CAD build for the part. Positions are in the model's coordinates, mm. A direction names the side the tool comes from. Give positions to 0.01 mm unless a question says otherwise; leave off trailing zeros. Write each loop counter-clockwise with the first axis right and the second up, starting at its lowest first coordinate (ties: lowest second). Pieces come first, ordered by that corner, then holes. Notation, with made-up numbers: (29.5, 68.25) - (81.5, 68.25) arc R23 ccw to (81.5, 104.25) - close; hole circle Ø7 at (69.25, -33). An arc over 180 degrees is marked (long way). Answer as a JSON object with one key per item and string values.
Autodesk Inventor part; units mm, degrees
ref_plane "YZ Plane" through (0, 0, 0) normal (1, 0, 0) x (0, 1, 0)
ref_plane "XZ Plane" through (0, 0, 0) normal (0, 1, 0) x (-1, 0, 0)
ref_plane "XY Plane" through (0, 0, 0) normal (0, 0, 1) x (1, 0, 0)
sketch "Sketch1" plane through (0, 0, 0) normal (1, 0, 0) x (0, 1, 0)
  line L0 (0, 9.5) -> (0, -9.5)
  line L1 (0, -9.5) -> (8, -9.5)
  line L2 (0, 9.5) -> (8, 9.5)
  line L3 (8, 9.5) -> (8, 14.5)
  line L4 (8, 14.5) -> (9.5, 14.5)
  line L5 (9.5, 14.5) -> (9.5, 10.5)
  line L6 (9.5, 10.5) -> (11.5, 10.5)
  line L7 (11.5, 10.5) -> (11.5, 16.5)
  line L8 (11.5, 16.5) -> (6, 16.5)
  line L9 (6, 16.5) -> (6, 11.5)
  line L10 (6, 11.5) -> (-3, 11.5)
  line L11 (-3, 11.5) -> (-4, 11.5)
  line L12 (-4, 11.5) -> (-4, 1)
  line L13 (0, 0) -> (3.5, 0)
  line L14 (0, -9.5) -> (8, -9.5)
  line L15 (8, -9.5) -> (8, -14.5)
  line L16 (8, -14.5) -> (9.5, -14.5)
  line L17 (9.5, -14.5) -> (9.5, -10.5)
  line L18 (11.5, -10.5) -> (11.5, -16.5)
  line L19 (11.5, -16.5) -> (6, -16.5)
  line L20 (6, -16.5) -> (6, -11.5)
  line L21 (6, -11.5) -> (-3, -11.5)
  line L22 (-3, -11.5) -> (-4, -11.5)
  line L23 (-4, -11.5) -> (-4, 1)
  line L24 (11.5, -10.5) -> (9.5, -10.5)
  point P0 (8.75, -16.5)
  point P1 (8.75, -14.5)
  dimension "d0" = 19
  dimension "d1" = 0
  dimension "d2" = 8
  dimension "d3" = 8
  dimension "d4" = 5
  dimension "d5" = 1.5
  dimension "d6" = 2
  dimension "d7" = 6
  dimension "d8" = 5.5
  dimension "d9" = 5
  dimension "d10" = 1
  dimension "d13" = 2
  dimension "d14" = 4
extrude "Extrusion1" add sketch "Sketch1" along normal blind 20
fillet "Fillet1" radius 5 2 edges at (10, 6, -11.5) (10, 6, 11.5)
chamfer "Chamfer1" distance 1 angle 45 12 edges at (20, 8, -12) (20, 8.75, -14.5) (20, 9.5, -12.5) (20, 8, 12) (20, 8.75, 14.5) (20, 9.5, 12.5) (0, 8, -12) (0, 8.75, -14.5) (0, 9.5, -12.5) (0, 8, 12) (0, 8.75, 14.5) (0, 9.5, 12.5)
sketch "Sketch2" plane through (0, 0, 9.5) normal (0, 1, 0) x (1, 0, 0)
  circle A0 centre (10, 9.5) radius 3
  line L0 (20, 19) -> (20, 0)
  line L1 (0, -7) -> (20, -7)
  point P0 (0, 9.5)
  dimension "d19" = 6
  dimension "d20" = 10
  dimension "d21" = 16.5
extrude "Extrusion2" cut sketch "Sketch2" against normal blind 20
chamfer "Chamfer2" distance 2.5 angle 45 1 edges at (7, 0, 0)
properties part number "Drziak_1"
(1) Saw through at D-D, the plane y = -1.5. Give the cut face in (x, z).
Answer key:
{"outline": "(0, -11.5) - (20, -11.5) - (20, 11.5) - (0, 11.5) - close; hole circle Ø8 at (10, 0)"}
(2) Pull direction Y, two halves, no side cores. Call faces 1 (the face through (10, 8, 12)), 2 (the face through (10.14, 4.5, 12.93)), 3 (the face through (10, 11, -10.5)): pulls with the +Y half, pulls with the -Y half, needs draft (parallel to the pull), parting line crosses it, or undercut.
Answer key:
{"face 1": "undercut", "face 2": "pulls with the -Y half", "face 3": "needs draft"}
(3) 3-axis set-ups, long thin cutter, end or side, ignore diameter. For faces 4 (the face through (0.5, 7.5, -12.5)), 5 (the face through (5, 0, 4)), 6 (the face through (10, -1, 11.5)), 7 (the face through (19.5, 7.5, -12.5)): which of +Z, -Z, +X, -X, +Y, -Y reach the whole face in a straight line?
Answer key:
{"face 4": "-X", "face 5": "+X, -X, +Y", "face 6": "+Z, +X, -X, -Y", "face 7": "+X"}
(4) Probe L1, parallel to Z at x = 9.75, y = 7.5; L2, parallel to X at y = -2.9, z = 0; L3, parallel to Z at x = 1.5, y = 10. List the from-to ranges inside material, lowest first. Write a range as [from, to].
Answer key:
{"L1": "z = [-16.5, -9.5], [9.5, 16.5]", "L2": "x = [0, 7], [13, 20]", "L3": "z = [-16.5, -10.5], [10.5, 16.5]"}
(5) Flat gauge pins, fed straight in: P1, Ø2.5, axis at x = 8, y = 4, coming from the -Z side; P2, Ø1.2, axis at x = 10, z = -12.5, coming from the -Y side; P3, Ø5.5, axis at x = 9, y = -2, coming from the -Z side. Where does each tip first touch, or does it go through?
Answer key:
{"P1": "stops at z = -13.87", "P2": "stops at y = 2.96", "P3": "stops at z = -11.5"}
(6) Saw through at B-B, the plane z = 0. Give the cut face in (x, y), and give its area (4 significant figures).
Answer key:
{"outline": "(0, -4) - (7, -4) - (7, -2.5) - (4.5, 0) - (0, 0) - close; (13, -4) - (20, -4) - (20, 0) - (15.5, 0) - (13, -2.5) - close", "area": "49.75 mm²"}
(7) Saw through at C-C, the plane y = 5. Give the cut face in (x, z), and give its area (3 significant figures).
Answer key:
{"outline": "(0, -13.5) - (20, -13.5) - (20, -9.5) - (0, -9.5) - close; (0, 9.5) - (20, 9.5) - (20, 13.5) - (0, 13.5) - close", "area": "160 mm²"}
